Verification items for the finished model (mm, model axes). Face numbers are marked on the shaded views. A direction names the side the tool comes from. Coordinates: 2 decimals unless noted, no trailing zeros. Loops run counter-clockwise (first coordinate to the right, second up) from the corner with the lowest first, then second, coordinate; pieces in that order, holes last.
Q1. Go/stop test with flat-tipped pins: P1, Ø1, axis at x = 1.5, y = -10, coming from the +Z side; P2, Ø5, axis at x = 3.5, z = 8.5, coming from the -Y side; P3, Ø2, axis at x = 3, z = -6.5, coming from the -Y side. Record where each tip stops, or that it passes through.
Q2. Sectioned sample at D-D (x = -4.25). Enter the section's corners in (y, z), then the cut area to 3 significant figures.
Q3. Mould release check, pull along Z, two halves, no side actions. Record for the marked faces 3, 4 and 5: +Z half, -Z half, draft (parallel to the pull), parting line (faces both ways), or undercut.
Q4. Sectioned sample at C-C (y = 12.75). Count the separate pieces of the cut face and the enclosed holes in it, then the cut area to 3 significant figures.
Q5. Access from +Z, -Z, +X, -X, +Y, -Y to the whole of each face (thin tool, end or side, straight path). Record for the marked faces 1 and 2.
Q6. Material ranges on probe 1 along Y at (x, z) = (0.5, 0); probe 2 along X at (y, z) = (4, -12); probe 3 along X at (y, z) = (13.75, 4.25), recorded low to high.
Q7. Sectioned sample at A-A (z = 0). Enter the section's corners in (x, y), then the cut area to 3 significant figures.
```python
from build123d import *

# Parameters (mm, degrees)
F_15_0_15_DURCHMESSER_BOHRUNG2_D = 15


with BuildPart() as part:
    # Skizze1 → Rotation1 (revolve)
    with BuildSketch(Plane.XY, mode=Mode.PRIVATE) as rotation1_sk:
        Polygon((-8.5, 0), (-8.5, 15), (-5, 12), (-1.5, 15), (1.5, 15), (5, 12), (8.5, 15), (8.5, 0), align=None)
    revolve(rotation1_sk.sketch.rotate(Axis((-85.191280049, 0, 0), (1, 0, 0)), 90), axis=Axis((-85.191280049, 0, 0), (1, 0, 0)))

    # Ø15.0 (15) Durchmesser Bohrung2 (through all)
    with Locations(Plane.ZY.offset(8.5)):
        with Locations((0, 0)):
            Hole(F_15_0_15_DURCHMESSER_BOHRUNG2_D / 2)


solid = part.part
```
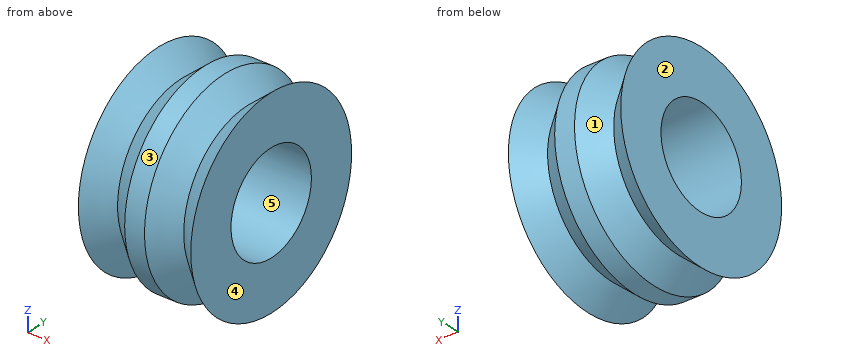
Geometry check:
1. P1: stops at z = 11.61
1. P2: stops at y = -13.27
1. P3: stops at y = -13.16
2. outline: circle Ø25.29 at (0, 0); hole circle Ø15 at (0, 0)
2. area: 325 mm2
3. face 3: parting line
3. face 4: draft
3. face 5: undercut
4. separate pieces: 3
4. enclosed holes: 0
4. area: 156 mm2
5. face 1: none
5. face 2: +Z, -Z, -X, +Y, -Y
6. probe 1: y = -15 to -7.5, 7.5 to 15
6. probe 2: x = -8.5 to -5.76, -4.24 to 4.24, 5.76 to 8.5
6. probe 3: x = -8.5 to -7.79, -2.21 to 2.21, 7.79 to 8.5
7. outline: (-8.5, -15) - (-5, -12) - (-1.5, -15) - (1.5, -15) - (5, -12) - (8.5, -15) - (8.5, -7.5) - (-8.5, -7.5) - close; (-8.5, 7.5) - (8.5, 7.5) - (8.5, 15) - (5, 12) - (1.5, 15) - (-1.5, 15) - (-5, 12) - (-8.5, 15) - close
7. area: 213 mm2
